from build123d import *

# Parameters (mm, degrees)
SKETCH1_R           = 6.9
SKETCH1_R_2         = 2.6
BOSS_EXTRUDE1_DEPTH = 10
BOSS_EXTRUDE2_DEPTH = 12
SKETCH3_R           = 7
SKETCH3_R_2         = 4
BOSS_EXTRUDE3_DEPTH = 4
BOSS_EXTRUDE4_DEPTH = 84
BOSS_EXTRUDE5_DEPTH = 84
CUT_EXTRUDE1_DEPTH  = 190.323263107
SCALE1_SCALE        = 1.5


with BuildPart() as part:
    # Sketch1 → Boss-Extrude1 (new body)
    with BuildSketch(Plane.XY):
        with BuildLine():
            Line((-155.070766667, -34.03543395), (-139.182010536, -34.03543395))
            Line((-139.182010536, -34.03543395), (-124.735717634, -34.03543395))
            add(Edge.make_bspline(
                [(-124.735717634, -34.03543395), (-120.868070652, -30.634901056), (-118.110731489, -25.337058748)],
                knots=[0.604913823, 0.604913823, 0.604913823, 1, 1, 1], degree=2))
            ThreePointArc((-118.110731489, -25.337058748), (-114.956411592, -18.057608365), (-121.224300514, -13.194101363))
            Line((-121.224300514, -13.194101363), (-122.374915538, -13.297224598))
            Line((-122.374915538, -13.297224598), (-145.504342678, -15.370186717))
            add(Edge.make_bspline(
                [(-145.504342678, -15.370186717), (-147.665446471, -15.751951197), (-150.237941893, -16.278752791)],
                knots=[0, 0, 0, 0.143499102, 0.143499102, 0.143499102], degree=2))
            add(Edge.make_bspline(
                [(-150.237941893, -16.278752791), (-156.331446907, -19.412430802), (-156.587305002, -28.504886835), (-155.070766667, -34.03543395)],
                knots=[0, 0, 0, 0, 1, 1, 1, 1], degree=3))
        make_face()
        with Locations((-142.777717077, -23.619181221)):
            Circle(SKETCH1_R, mode=Mode.SUBTRACT)
        with Locations((-121.224300514, -19.664754316)):
            Circle(SKETCH1_R_2, mode=Mode.SUBTRACT)
    boss_extrude1 = extrude(amount=BOSS_EXTRUDE1_DEPTH)

    # Sketch2 → Boss-Extrude2 (add)
    with BuildSketch(Plane(origin=(0, 0, 0), x_dir=(-1, 0, 0), z_dir=(0, 0, -1))):
        with BuildLine():
            Line((124.810828249, -34.03543395), (124.810828249, -33.03543395))
            ThreePointArc((124.810828249, -33.03543395), (125.396614687, -31.621220388), (126.810828249, -31.03543395))
            Line((126.810828249, -31.03543395), (155.660238601, -31.03543395))
            add(Edge.make_bspline(
                [(155.660238601, -31.03543395), (155.453340821, -32.220849379), (155.070766667, -34.03543395)],
                knots=[0.469279702, 0.469279702, 0.469279702, 1.113861257, 1.113861257, 1.113861257], degree=2))
            Line((155.070766667, -34.03543395), (124.810828249, -34.03543395))
        make_face()
    extrude(amount=BOSS_EXTRUDE2_DEPTH)

    # Mirror1: Boss-Extrude1 across plane
    add(boss_extrude1.mirror(Plane(origin=(0, 0, -6), x_dir=(1, 0, 0), z_dir=(0, 0, -1))))

    # Sketch3 → Boss-Extrude3 (add)
    with BuildSketch(Plane(origin=(0, 0, 0), x_dir=(-1, 0, 0), z_dir=(0, 0, -1))):
        with Locations((142.777717077, -23.619181221)):
            Circle(SKETCH3_R)
        with Locations((142.777717077, -23.619181221)):
            Circle(SKETCH3_R_2, mode=Mode.SUBTRACT)
    boss_extrude3 = extrude(amount=-BOSS_EXTRUDE3_DEPTH)

    # Mirror2: Boss-Extrude3 across plane
    add(boss_extrude3.mirror(Plane(origin=(0, 0, -6), x_dir=(1, 0, 0), z_dir=(0, 0, -1))))

    # Sketch4 → Boss-Extrude4 (add)
    with BuildSketch(Plane.XY.offset(10)):
        with BuildLine():
            add(Edge.make_bspline(
                [(-155.660238601, -31.03543395), (-155.52477055, -32.104378324), (-155.322110933, -33.11882586), (-155.070766667, -34.03543395)],
                knots=[0.834264482, 0.834264482, 0.834264482, 0.834264482, 1, 1, 1, 1], degree=3))
            Line((-155.070766667, -34.03543395), (-124.735717634, -34.03543395))
            add(Edge.make_bspline(
                [(-124.735717634, -34.03543395), (-123.199822379, -32.685036057), (-121.8390218, -31.03543395)],
                knots=[0, 0, 0, 1, 1, 1], degree=2))
            Line((-121.8390218, -31.03543395), (-155.660238601, -31.03543395))
        make_face()
    extrude(amount=BOSS_EXTRUDE4_DEPTH)

    # Sketch5 → Boss-Extrude5 (add)
    with BuildSketch(Plane(origin=(0, 0, -22), x_dir=(-1, 0, 0), z_dir=(0, 0, -1))):
        with BuildLine():
            Line((155.070766667, -34.03543395), (124.735717633, -34.035433949))
            add(Edge.make_bspline(
                [(124.735717633, -34.035433949), (123.199822378, -32.685036056), (121.8390218, -31.03543395)],
                knots=[0, 0, 0, 1, 1, 1], degree=2))
            Line((121.8390218, -31.03543395), (155.660238601, -31.03543395))
            add(Edge.make_bspline(
                [(155.660238601, -31.03543395), (155.52477055, -32.104378324), (155.322110933, -33.11882586), (155.070766667, -34.03543395)],
                knots=[0.834264482, 0.834264482, 0.834264482, 0.834264482, 1, 1, 1, 1], degree=3))
        make_face()
    extrude(amount=BOSS_EXTRUDE5_DEPTH)

    # Sketch6 → Cut-Extrude1 (cut, through all)
    with BuildSketch(Plane(origin=(0, -31.03543395, 0), x_dir=(1, 0, 0), z_dir=(0, 1, 0))):
        Polygon((-137.786415389, 76.894835229), (-142.400005748, 77.114191864), (-144.516832509, 81.219356636), (-142.02006891, 85.105164771), (-137.406478551, 84.885808136), (-135.289651791, 80.780643364), align=None)
        Polygon((-135.289651791, 30.780643364), (-137.786415389, 26.894835229), (-142.400005748, 27.114191864), (-144.516832509, 31.219356636), (-142.02006891, 35.105164771), (-137.406478551, 34.885808136), align=None)
        with BuildLine():
            Line((-155.6602386, 22), (-173.465321409, 22))
            Line((-173.465321409, 22), (-173.465321409, 117.834139367))
            Line((-173.465321409, 117.834139367), (-100.430925903, 117.834139367))
            Line((-100.430925903, 117.834139367), (-121.8390218, 22))
            add(Edge.make_bspline(
                [(-121.8390218, 22), (-130.237957541, 29.288236007), (-131.708688401, 51.819501052), (-127.475857655, 72.230953717), (-131.071963897, 82.863468574)],
                knots=[0, 0, 0, 0, 0.490729359, 1, 1, 1, 1], degree=3))
            ThreePointArc((-131.071963897, 82.863468574), (-140.840035974, 89.976993263), (-148.928982602, 81))
            add(Edge.make_bspline(
                [(-148.928982602, 81), (-152.625386512, 74.081760345), (-155.262352814, 54.105117148), (-154.402874629, 34.24459948), (-155.6602386, 22)],
                knots=[0, 0, 0, 0, 0.385424941, 1, 1, 1, 1], degree=3))
        make_face()
        with BuildLine():
            Line((-100.430925903, -105.834139367), (-121.8390218, -10))
            add(Edge.make_bspline(
                [(-121.8390218, -10), (-130.237957541, -17.288236007), (-131.708688401, -39.819501052), (-127.475857655, -60.230953717), (-131.071963897, -70.863468574)],
                knots=[0, 0, 0, 0, 0.490729359, 1, 1, 1, 1], degree=3))
            ThreePointArc((-131.071963897, -70.863468574), (-140.840035974, -77.976993263), (-148.928982602, -69))
            add(Edge.make_bspline(
                [(-148.928982602, -69), (-152.625386512, -62.081760345), (-155.262352814, -42.105117148), (-154.402874629, -22.24459948), (-155.6602386, -10)],
                knots=[0, 0, 0, 0, 0.385424941, 1, 1, 1, 1], degree=3))
            Line((-155.6602386, -10), (-173.465321409, -10))
            Line((-173.465321409, -10), (-173.465321409, -105.834139367))
            Line((-173.465321409, -105.834139367), (-100.430925903, -105.834139367))
        make_face()
        Polygon((-142.02006891, -23.105164771), (-137.406478551, -22.885808136), (-135.289651791, -18.780643364), (-137.786415389, -14.894835229), (-142.400005748, -15.114191864), (-144.516832509, -19.219356636), align=None)
        Polygon((-135.289651791, -68.780643364), (-137.786415389, -64.894835229), (-142.400005748, -65.114191864), (-144.516832509, -69.219356636), (-142.02006891, -73.105164771), (-137.406478551, -72.885808136), align=None)
    extrude(amount=-CUT_EXTRUDE1_DEPTH, mode=Mode.SUBTRACT)


with BuildPart() as part_1:
    # Scale1: scaled about (-137.903774464, -28.080076636, -5.999999982)
    add(part.part.scale(SCALE1_SCALE).moved(Location((68.951887232, 14.040038318, 2.999999991))))


solid = part_1.part
Verification items for the finished model (mm, model axes). A direction names the side the tool comes from. Give positions to 0.01 mm unless a question says otherwise; leave off trailing zeros. Write item = value, one per line.
(1) Go/stop test with flat-tipped pins: pin 1 Ø9 at (x, y) = (-112.88, -15.46) entering from +Z; pin 2 Ø9.5 at (x, y) = (-145.21, -21.39) entering from -Z; pin 3 Ø10.5 at (x, y) = (-148.5, -19.5) entering from -Z; pin 4 Ø20 at (x, z) = (-151.5, -7) entering from +Y. Record where each tip stops, or that it passes through.
Found:
pin_1 = 18
pin_2 = through
pin_3 = -21
pin_4 = -8.67
(2) Access from +Z, -Z, +X, -X, +Y, -Y to the whole of each face (thin tool, end or side, straight path). Record for faces 4 (the face through (-109.165, -14.286, -22.395)), 5 (the face through (-140.666, -34.732, 112.496)), 6 (the face through (-144, -32.513, -80)), 7 (the face through (-103.44, -13.22, 10.39)), 8 (the face through (-150, -26, -21)).
Found:
face_4 = +Z, -Z
face_5 = +Y, -Y
face_6 = -Z, +X, -X, +Y
face_7 = +Z, -Z, +X
face_8 = -Z
(3) Material ranges on line 1 (Z direction, x = -119, y = -10.5); line 2 (Z direction, x = -146, y = -30); line 3 (Y direction, x = -157, z = -35), recorded low to high.
Found:
line_1 = -30 to -15, 3 to 18
line_2 = -21 to -15, 3 to 9
line_3 = -37.01 to -32.51
(4) Draft check along Z on faces 1 (the face through (-134.8, -18.9, 18)), 2 (the face through (-134.8, -18.9, -30)), 3 (the face through (-140.666, -34.732, 37.496)). Enter one of: released by +Z, released by -Z, zero draft, split by the parting line, or undercut.
Found:
face_1 = released by +Z
face_2 = released by -Z
face_3 = undercut
